Autodesk Inventor part; units mm, degrees
ref_plane "YZ Plane" through (0, 0, 0) normal (1, 0, 0) x (0, 1, 0)
ref_plane "XZ Plane" through (0, 0, 0) normal (0, 1, 0) x (-1, 0, 0)
ref_plane "XY Plane" through (0, 0, 0) normal (0, 0, 1) x (1, 0, 0)
sketch "Sketch1" plane through (0, 0, 0) normal (0, 0, 1) x (1, 0, 0)
  circle A0 centre (0, 0) radius 31.75
  circle A1 centre (0, 0) radius 34.798
  circle A2 centre (0, 0) radius 41.402
  line L0 (-46.482, 46.482) -> (46.482, 46.482)
  line L1 (46.482, 46.482) -> (46.482, -46.482)
  line L2 (46.482, -46.482) -> (-46.482, -46.482)
  line L3 (-46.482, -46.482) -> (-46.482, 46.482)
  line L4 (0, 46.482) -> (0, 41.402) construction
  line L5 (0, -41.402) -> (0, -46.482) construction
  line L6 (-46.482, 0) -> (-41.402, 0) construction
  line L7 (46.482, 0) -> (41.402, 0) construction
  dimension "d0" = 63.5
  dimension "d1" = 69.596
  dimension "d2" = 82.804
  dimension "d3" = 5.08
extrude "Extrusion1" add sketch "Sketch1" along normal blind 5.08 contours A1 | A2 | L0 L1 L2 L3
extrude "Extrusion2" add sketch "Sketch1" along normal blind 19.05 contours A1
extrude "Extrusion3" add sketch "Sketch1" along normal blind 19.05 contours L0 L1 L2 L3
sketch "Sketch2" plane through (0, 0, 0) normal (0, 0, -1) x (-1, 0, 0)
  circle A0 centre (0, 0) radius 34.798 construction
  line L0 (46.482, 46.482) -> (-46.482, 46.482)
  line L1 (-5.3975, 46.482) -> (5.3975, 46.482)
  line L2 (5.3975, 46.482) -> (5.3975, 36.068)
  line L3 (5.3975, 36.068) -> (-5.3975, 36.068)
  line L4 (-5.3975, 36.068) -> (-5.3975, 46.482)
  line L5 (0, 34.798) -> (0, 36.068) construction
  dimension "d10" = 10.795
  dimension "d11" = 1.27
extrude "Extrusion4" cut sketch "Sketch2" against normal blind 19.05
chamfer "Chamfer1" distance 19.05 angle 45 2 edges at (46.482, 46.482, 9.525) (-46.482, 46.482, 9.525)
fillet "Fillet1" radius 3.175 8 edges at (46.482, -46.482, 9.525) (46.482, 27.432, 9.525) (27.432, 46.482, 9.525) (5.3975, 46.482, 9.525) (-5.3975, 46.482, 9.525) (-27.432, 46.482, 9.525) (-46.482, 27.432, 9.525) (-46.482, -46.482, 9.525)
sketch "Sketch3" plane through (0, 0, 0) normal (0, 0, -1) x (-1, 0, 0)
  circle A0 centre (0, 0) radius 31.75
  circle A1 centre (0, 0) radius 4.1275
  dimension "d18" = 8.255
extrude "Extrusion5" add sketch "Sketch3" against normal blind 4.445
fillet "Fillet2" radius 6.35 1 edges at (-31.75, 0, 4.445)
properties part number "BallastTankMillFixture"
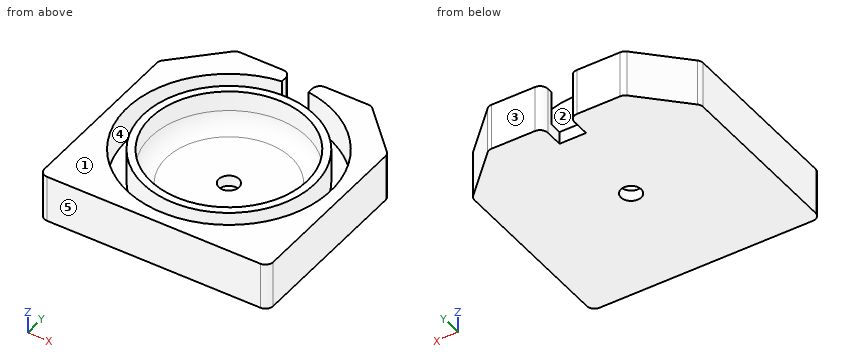
Geometry check sheet. Reference: the model listing, model coordinates, mm. Face numbers are marked on the shaded views. A direction names the side the tool comes from. Coordinates: 2 decimals unless noted, no trailing zeros. Answer as a JSON object with one key per item and string values. Group by question number.
Item 1: Draft check along Y on the marked faces 1, 2 and 3. Enter one of: +Y half, -Y half, draft (parallel to the pull), parting line (faces both ways), or undercut.
Item 2: Sectioned sample at A-A, the plane z = 17. Give the number of separate pieces and of enclosed holes in the cut face, and give its area (3 significant figures).
Item 3: Scan lines: probe 1 along Y at (x, z) = (0, 14.5); probe 2 along Y at (x, z) = (0, 2.6); probe 3 along X at (y, z) = (8.5, 9). Record each from-to range of solid material in increasing order.
Item 4: Depth check by flat-ended pin: pin 1 Ø8 at (y, z) = (38, 6.5) entering from -X; pin 2 Ø8 at (x, z) = (-0.5, 8) entering from +Y; pin 3 Ø10 at (x, z) = (-32.5, 16) entering from +Y. Enter the tip coordinate at first touch or a pass-through.
Item 5: Tool access check on the marked faces 4 and 5. Record the directions out of +Z, -Z, +X, -X, +Y, -Y that give a thin tool (end or side, any length) a straight path to the whole face; none if there is none.
Resolved:
{
 "1": {"face 1": "draft", "face 2": "undercut", "face 3": "+Y half"},
 "2": {"separate pieces": "2", "enclosed holes": "1", "area": "3,470 mm^2"},
 "3": {"probe 1": "-46.48 to -41.4, -34.8 to -31.75, 31.75 to 34.8", "probe 2": "-46.48 to -4.13, 4.13 to 36.07", "probe 3": "-46.48 to -40.52, -33.74 to -30.32, 30.32 to 33.74, 40.52 to 46.48"},
 "4": {"pin 1": "x = -39.91", "pin 2": "y = 36.07", "pin 3": "y = 46.16"},
 "5": {"face 4": "+Z", "face 5": "+Z, -Z, +X, -X, -Y"}
}
